The drawing under review shows one solid part. Ordinate dimensions are in mm from its lowest x, y, z. Coordinates: 2 decimals unless noted, no trailing zeros. Order: outer loops, then holes, each group sorted by start corner. A loop starts at its lowest first (then second) coordinate and runs counter-clockwise, first axis right, second up.
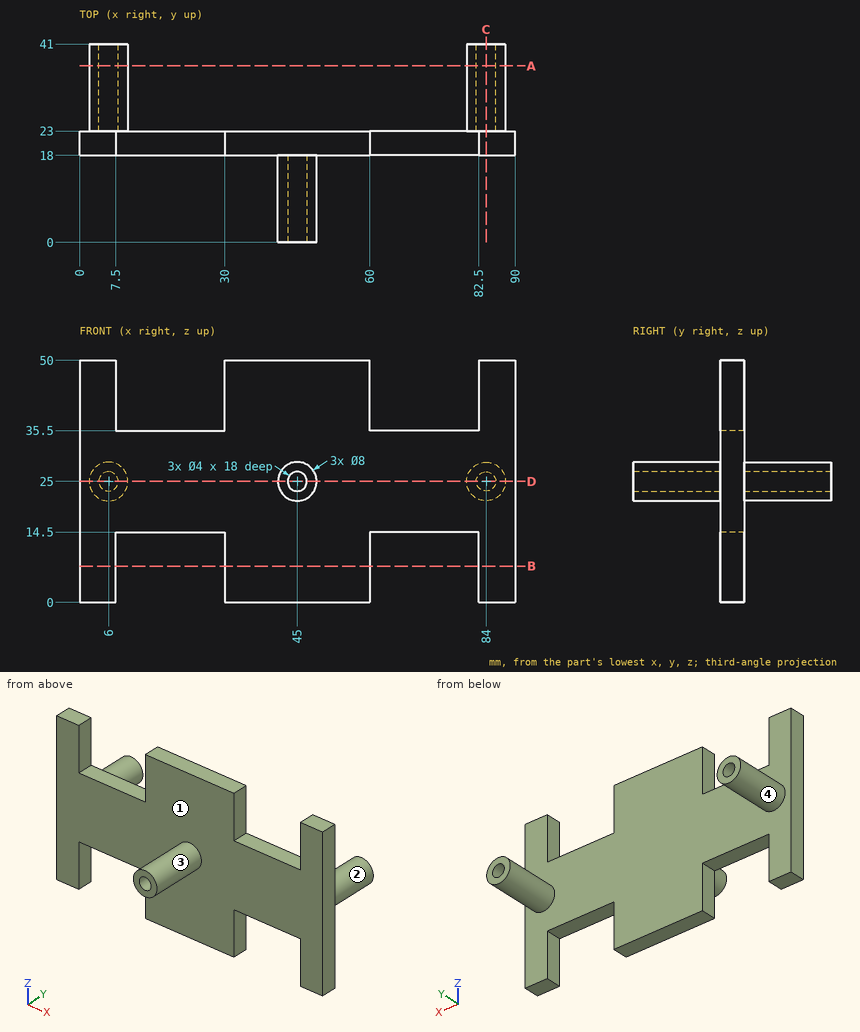
1. Clearance check with flat-ended pins moving along their axes: pin 1 Ø3 at (x, z) = (64.5, 20) entering from -Y; pin 2 Ø4 at (x, y) = (22, 21) entering from -Z; pin 3 Ø1.2 at (x, z) = (6.5, 26) entering from +Y. State where each tip first meets the part, or that it passes through.
Answer below:
pin 1: stops at y = 18
pin 2: stops at z = 14.5
pin 3: stops at y = 23
2. Take a section at D-D, the plane z = 25. Give the boundary of the cut face in (x, y), plus the area to 3 significant figures.
Answer below:
outline: (0, 18) - (41, 18) - (41, 0) - (43, 0) - (43, 18) - (47, 18) - (47, 0) - (49, 0) - (49, 18) - (90, 18) - (90, 23) - (88, 23) - (88, 41) - (86, 41) - (86, 23) - (82, 23) - (82, 41) - (80, 41) - (80, 23) - (10, 23) - (10, 41) - (8, 41) - (8, 23) - (4, 23) - (4, 41) - (2, 41) - (2, 23) - (0, 23) - close
area: 666 mm2
3. To check wall thickness, follow L1, parallel to X at y = 31.25, z = 25; L2, parallel to X at y = 21, z = 47.5; L3, parallel to X at y = 4, z = 25. State the ranges of each line that lie inside material, in increasing order.
Answer below:
L1: x = 2 to 4, 8 to 10, 80 to 82, 86 to 88
L2: x = 0 to 7.5, 30 to 60, 82.5 to 90
L3: x = 41 to 43, 47 to 49
4. Take a section at A-A, the plane y = 36.5. Give the boundary of the cut face in (x, z), plus the area to 3 significant figures.
Answer below:
outline: circle Ø8 at (6, 25); circle Ø8 at (84, 25); hole circle Ø4 at (6, 25); hole circle Ø4 at (84, 25)
area: 75.4 mm2
5. Take a section at B-B, the plane z = 7.5. Give the boundary of the cut face in (x, y), plus the area to 3 significant figures.
Answer below:
outline: (0, 18) - (7.5, 18) - (7.5, 23) - (0, 23) - close; (30, 18) - (60, 18) - (60, 23) - (30, 23) - close; (82.5, 18) - (90, 18) - (90, 23) - (82.5, 23) - close
area: 225 mm2
6. Take a section at C-C, the plane x = 84. Give the boundary of the cut face in (y, z).
Answer below:
outline: (18, 0) - (23, 0) - (23, 21) - (41, 21) - (41, 23) - (23, 23) - (23, 27) - (41, 27) - (41, 29) - (23, 29) - (23, 50) - (18, 50) - close
7. The part is to be moulded in two halves that separate along X. For the marked faces 1, 2, 3 and 4, say which applies: +X half, -X half, draft (parallel to the pull), parting line (faces both ways), or undercut.
Answer below:
face 1: draft
face 2: undercut
face 3: parting line
face 4: undercut
